Check sheet for the drawn part. Datum: minimum x, y, z corner. Units: mm. A direction names the side the tool comes from. Coordinates: 2 decimals unless noted, no trailing zeros. Write each loop counter-clockwise with the first axis right and the second up, starting at its lowest first coordinate (ties: lowest second). Pieces come first, ordered by that corner, then holes. Notation, with made-up numbers: M 43,11 L 74,11 A19 ccw 74,48 Z; hole C 49.25,9.25 d2. An arc over 180 degrees is marked long. Answer in a Markdown table with one row per item.
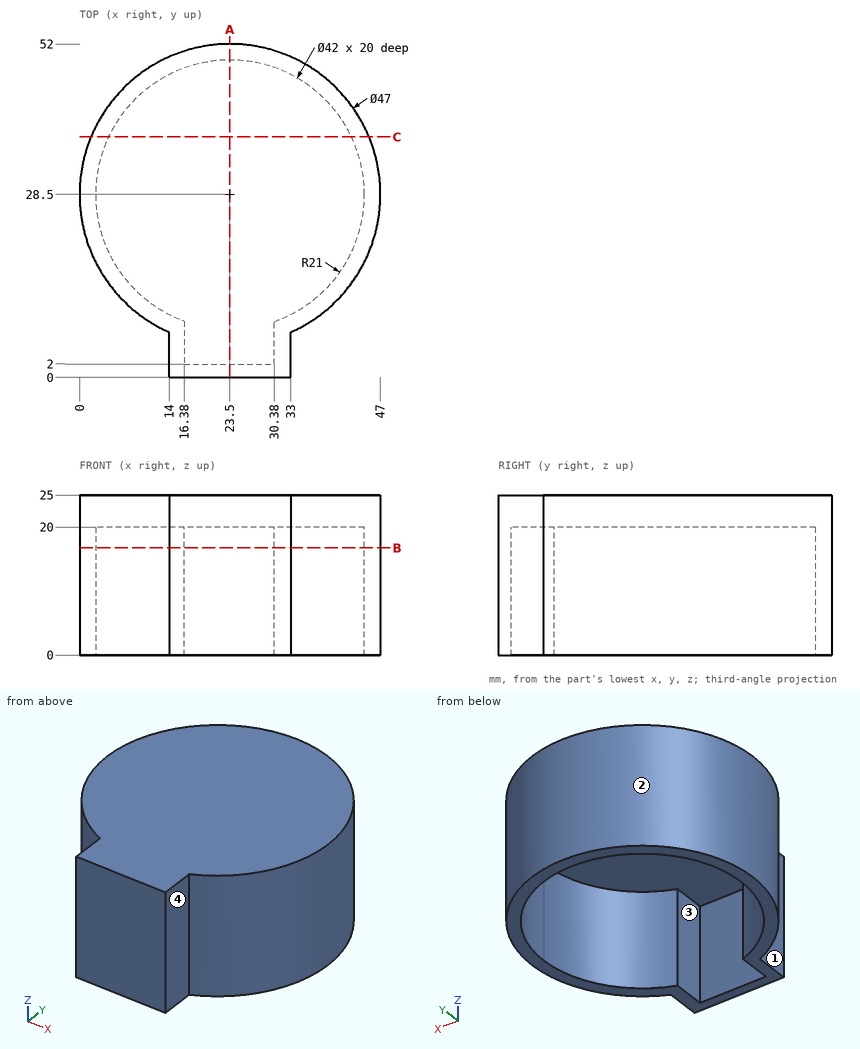
1) Thickness scan on L1, parallel to X at y = 28.5, z = 15; L2, parallel to Y at x = 23.5, z = 13.25; L3, parallel to X at y = 4, z = 14.75. Record the ranges inside material, lowest first. Write a range as [from, to].
Response values:
| item | result |
|---|---|
| L1 | x = [0, 2.5], [44.5, 47] |
| L2 | y = [0, 2], [49.5, 52] |
| L3 | x = [14, 16.38], [30.38, 33] |
2) Depth check by flat-ended pin: pin 1 (3 mm diameter, centred on y = 10, z = 6.5, fed in from +X) (1 decimal); pin 2 (3.5 mm diameter, centred on y = 6, z = 8, fed in from -X); pin 3 (5 mm diameter, centred on x = 11.5, y = 16, fed in from -Z); pin 4 (10 mm diameter, centred on x = 20.5, z = 14.5, fed in from +Y). Enter the tip coordinate at first touch or a pass-through.
Response values:
| item | result |
|---|---|
| pin 1 | stops at x = 39.7 |
| pin 2 | stops at x = 12.47 |
| pin 3 | stops at z = 20 |
| pin 4 | stops at y = 52 |
3) Tool access check on the marked faces 1, 2, 3 and 4. Record the directions out of +Z, -Z, +X, -X, +Y, -Y that give a thin tool (end or side, any length) a straight path to the whole face; none if there is none.
Response values:
| item | result |
|---|---|
| face 1 | +Z, -Z, -X, -Y |
| face 2 | +Z, -Z |
| face 3 | -Z |
| face 4 | +Z, -Z, +X, -Y |
4) Sectioned sample at B-B (z = 16.75). Record the cut outline in (x, y).
Response values:
| item | result |
|---|---|
| outline | M 14,0 L 33,0 L 33,7.01 A23.5 ccw long 14,7.01 Z; hole M 16.38,2 L 30.38,2 L 30.38,8.66 A21 ccw long 16.38,8.74 Z |
5) Sectioned sample at C-C (y = 37.5). Record the cut outline in (x, z).
Response values:
| item | result |
|---|---|
| outline | M 1.79,0 L 4.53,0 L 4.53,20 L 42.47,20 L 42.47,0 L 45.21,0 L 45.21,25 L 1.79,25 Z |
6) Sectioned sample at A-A (x = 23.5). Record the cut outline in (y, z), then the cut area to 3 significant figures.
Response values:
| item | result |
|---|---|
| outline | M 0,0 L 2,0 L 2,20 L 49.5,20 L 49.5,0 L 52,0 L 52,25 L 0,25 Z |
| area | 350 mm² |
